Verification items for the finished model (mm, model axes). Round coordinates to 2 decimals unless told otherwise and drop trailing zeros. Write each loop counter-clockwise with the first axis right and the second up, starting at its lowest first coordinate (ties: lowest second). Pieces come first, ordered by that corner, then holes. Notation, with made-up numbers: M 14.25,73 L 38.25,73 A13 cw 38.25,94 Z; hole C -14,15 d2. An arc over 180 degrees is marked long. Answer in a Markdown table with one row per item. Add a question column.
1. Material ranges on probe 1 along Z at (x, y) = (-69.85, -32.75); probe 2 along X at (y, z) = (-33, -139); probe 3 along Z at (x, y) = (-69, -34), recorded low to high.
2. Sectioned sample at A-A on z = 31. Record the cut outline in (x, y), plus the area to 3 significant figures.
3. Go/stop test with flat-tipped pins: pin 1 Ø1 at (x, z) = (20.5, -142.5) entering from +Y; pin 2 Ø5.5 at (x, z) = (-69.85, 12.7) entering from -Y; pin 3 Ø5 at (x, z) = (69.85, 165.1) entering from +Y; pin 4 Ø6.5 at (x, z) = (-70.5, 13) entering from -Y. Record where each tip stops, or that it passes through.
4. Sectioned sample at C-C on z = 180. Record the cut outline in (x, y), plus the area to 3 significant figures.
5. Sectioned sample at B-B on x = 36. Record the cut outline in (y, z), plus the area to 3 significant figures.
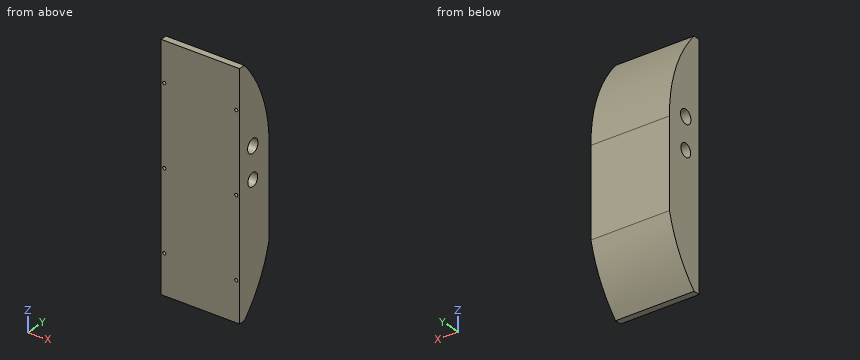
Autodesk Inventor part; units mm, degrees
ref_plane "YZ Plane" through (0, 0, 0) normal (1, 0, 0) x (0, 1, 0)
ref_plane "XZ Plane" through (0, 0, 0) normal (0, 1, 0) x (-1, 0, 0)
ref_plane "XY Plane" through (0, 0, 0) normal (0, 0, 1) x (1, 0, 0)
sketch "Sketch1" plane through (0, 0, 0) normal (1, 0, 0) x (0, 1, 0)
  line L0 (-38.1, -165.1) -> (-38.1, 165.1)
  line L1 (-38.1, 165.1) -> (20.949, 165.1)
  line L2 (38.1, 77.5498) -> (38.1, -100.5752)
  line L3 (12.4566, -165.1) -> (-38.1, -165.1)
  line L4 (-38.1, -165.1) -> (38.1, 165.1) construction
  line L5 (-38.1, 165.1) -> (38.1, -165.1) construction
  line L6 (-38.1, -165.1) -> (-38.1, -215.9)
  line L7 (-38.1, -215.9) -> (-25.4, -215.9)
  line L8 (-25.4, -215.9) -> (-25.4, -165.1)
  line L9 (-38.1, 165.1) -> (-38.1, 241.3)
  line L10 (-38.1, 241.3) -> (-25.4, 241.3)
  line L11 (-25.4, 241.3) -> (-25.4, 165.1)
  line L12 (-38.1, -139.7) -> (38.1, -139.7) construction
  line L13 (-38.1, 12.7) -> (38.1, 12.7) construction
  line L14 (-38.1, 165.1) -> (38.1, 165.1) construction
  arc A0 (38.1, 68.9574) -> (-25.4, 241.3) centre (-215.8637, 73.2536) ccw
  arc A1 (-25.4, -215.9) -> (38.1, -100.5752) centre (-208.549, -39.9101) ccw
  point P0 (0, 0)
  dimension "d0" = 330.2
  dimension "d1" = 76.2
  dimension "d2" = 50.8
  dimension "d3" = 12.7
  dimension "d5" = 76.2
  dimension "d6" = 12.7
  dimension "d9" = 152.4
  dimension "d10" = 76.2
  dimension "d11" = 152.4
  dimension "d37" = 254
  dimension "d38" = 254
extrude "Extrusion1" add sketch "Sketch1" along normal mid plane 152.4
sketch "Sketch3" plane through (-76.2, -38.1, -215.9) normal (0, -1, 0) x (1, 0, 0)
  circle A0 centre (6.35, 76.2) radius 2.9972
  line L0 (0, 0) -> (0, 457.2)
  line L1 (0, 0) -> (152.4, 0)
  circle A1 centre (146.05, 76.2) radius 2.9972
  circle A2 centre (6.35, 228.6) radius 2.9972
  circle A3 centre (146.05, 228.6) radius 2.9972
  circle A4 centre (6.35, 381) radius 2.9972
  circle A5 centre (146.05, 381) radius 2.9972
  point P0 (76.2, 215.9)
  dimension "d14" = 5.9944
  dimension "d15" = 6.35
  dimension "d16" = 76.2
  dimension "d19" = 139.7
  dimension "d22" = 152.4
extrude "Extrusion2" cut sketch "Sketch3" against normal blind 12.7
ref_plane "Work Plane1" through (0, 0, 0) normal (1, 0, 0) x (0, 0, -1)
sketch "Sketch5" plane through (-76.2, 0, 0) normal (-1, 0, 0) x (0, 0, 1)
  circle A0 centre (87.0752, -3.8046) radius 13.462
  point P0 (0, 0)
extrude "Extrusion4" cut sketch "Sketch5" against normal through all
sketch "Sketch6" plane through (-76.2, 0, 0) normal (-1, 0, 0) x (0, 0, 1)
  circle A0 centre (26.9178, -3.8046) radius 12.7
  point P0 (0, 0)
  dimension "d41" = 25.4
extrude "Extrusion5" cut sketch "Sketch6" against normal through all
properties part number "WingBox"
Geometry check:
| question | item | result |
|---|---|---|
| 1 | probe 1 | z = -215.9 to -142.7, -136.7 to 9.7, 15.7 to 162.1, 168.1 to 241.3 |
| 1 | probe 2 | x = -76.2 to -72.76, -66.94 to 66.94, 72.76 to 76.2 |
| 1 | probe 3 | z = -215.9 to -142.57, -136.83 to 9.83, 15.57 to 162.23, 167.97 to 241.3 |
| 2 | outline | M -76.2,-38.1 L 76.2,-38.1 L 76.2,-15.83 L -76.2,-15.83 Z; M -76.2,8.22 L 76.2,8.22 L 76.2,38.1 L -76.2,38.1 Z |
| 2 | area | 7,950 mm2 |
| 3 | pin 1 | stops at y = 24.03 |
| 3 | pin 2 | stops at y = -25.4 |
| 3 | pin 3 | stops at y = 21.9 |
| 3 | pin 4 | stops at y = -38.1 |
| 4 | outline | M -76.2,-38.1 L 76.2,-38.1 L 76.2,14.62 L -76.2,14.62 Z |
| 4 | area | 8,030 mm2 |
| 5 | outline | M -38.1,-215.9 L -25.4,-215.9 A254 ccw 38.1,-100.58 L 38.1,68.96 A254 ccw -25.4,241.3 L -38.1,241.3 Z; hole C -3.8,87.08 d26.92; hole C -3.8,26.92 d25.4 |
| 5 | area | 27,500 mm2 |
